Here's the drawing with two shaded views (mm, measured from the low corner). I have some questions. Round coordinates to 2 decimals unless told otherwise and drop trailing zeros. Loops run counter-clockwise (first coordinate to the right, second up) from the corner with the lowest first, then second, coordinate; pieces in that order, holes last.
(1) If I drill on line 1 along Z through (x, y) = (0.6, 82); line 2 along Y through (x, z) = (2.75, 8.5); line 3 along Y through (x, z) = (1.3, 6.5), over which ranges is the centre line in solid material (lowest first)?
(2) I want a section at D-D on z = 8. Write out the boundary of the cut face in (x, y).
(3) I want a section at C-C on y = 92. Write out the boundary of the cut face in (x, z), plus the area to 3 significant figures.
(4) I want a section at A-A on z = 16. Write out the boundary of the cut face in (x, y), plus the area to 3 significant figures.
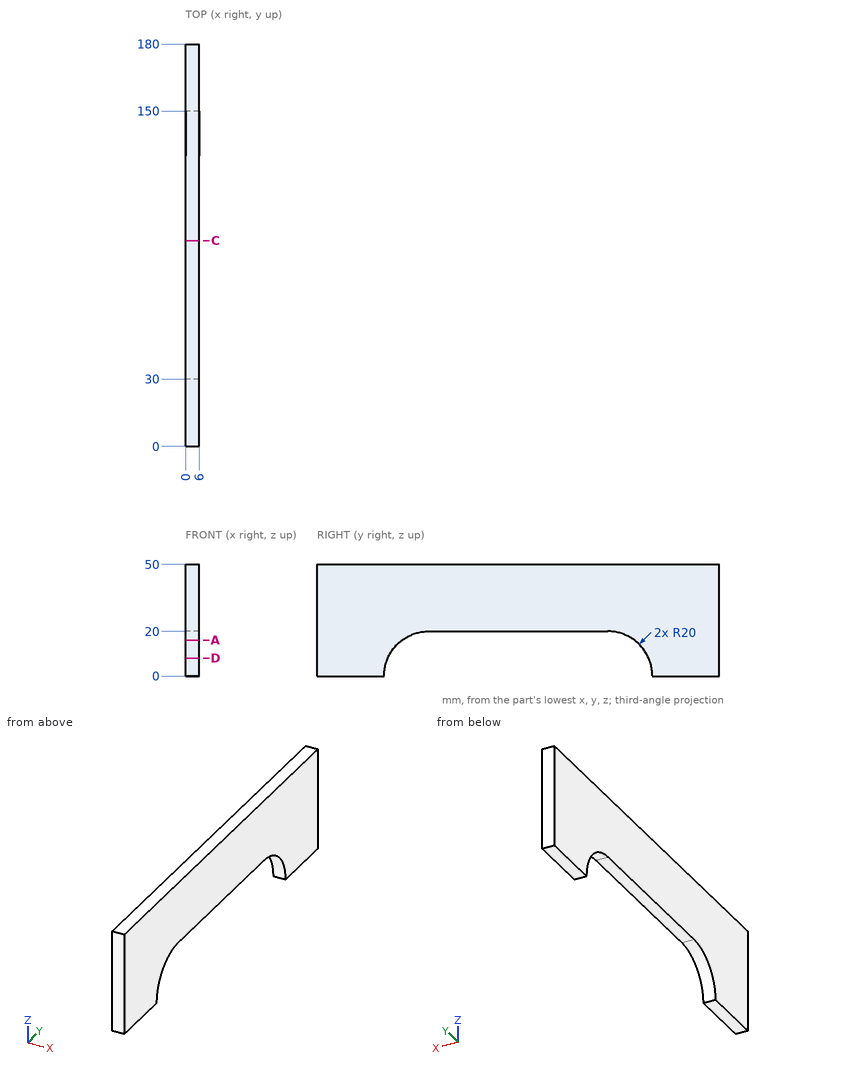
Filled sheet:
1. line 1: z = 20 to 50
1. line 2: y = 0 to 31.9, 148.1 to 180
1. line 3: y = 0 to 31.09, 148.91 to 180
2. outline: (0, 0) - (6, 0) - (6, 31.67) - (0, 31.67) - close; (0, 148.33) - (6, 148.33) - (6, 180) - (0, 180) - close
3. outline: (0, 20) - (6, 20) - (6, 50) - (0, 50) - close
3. area: 180 mm2
4. outline: (0, 0) - (6, 0) - (6, 38) - (0, 38) - close; (0, 142) - (6, 142) - (6, 180) - (0, 180) - close
4. area: 456 mm2
